Verification items for the finished model (mm, model axes). Coordinates: 2 decimals unless noted, no trailing zeros. Order: outer loops, then holes, each group sorted by start corner. A loop starts at its lowest first (then second) coordinate and runs counter-clockwise, first axis right, second up.
Q1. Thickness scan on line 1 (X direction, y = 177.8, z = 1.8); line 2 (Y direction, x = 12.7, z = 0.9); line 3 (Y direction, x = 495.3, z = 2.05). Record the ranges inside material, lowest first.
Q2. Depth check by flat-ended pin: P1, Ø3, axis at x = 57.15, y = 12.7, coming from the -Z side (3 decimals); P2, Ø1.6, axis at x = 207, z = 1.5, coming from the -Y side. Enter the tip coordinate at first touch or a pass-through.
Q3. Cross-section at B-B, the plane z = 1.6. Count the separate pieces of the cut face and the enclosed holes in it, and give its area (3 significant figures).
Q4. Cross-section at C-C, the plane y = 193. Record the boundary of the cut face in (x, z) (3 decimals).
Q5. Cross-section at D-D, the plane x = 223.5. Record the boundary of the cut face in (y, z) (3 decimals), and give its area (3 significant figures).
from build123d import *

# Parameters (mm, degrees)
SKETCH1_W           = 508
SKETCH1_H           = 508
BOSS_EXTRUDE1_DEPTH = 3.175
SKETCH2_R           = 2.54
SKETCH2_W           = 234.95
SKETCH2_H           = 368.3
CUT_EXTRUDE1_DEPTH  = 44.45
SKETCH4_R           = 2.159
CUT_EXTRUDE3_DEPTH  = 719.427505476
SKETCH5_R           = 2.6
CUT_EXTRUDE4_DEPTH  = 719.427505476
SKETCH6_W           = 487.3625
SKETCH6_H           = 76.2
CUT_EXTRUDE5_DEPTH  = 719.427505476


with BuildPart() as part:
    # Sketch1 → Boss-Extrude1 (new body)
    with BuildSketch(Plane.XY):
        with Locations((254, 254)):
            Rectangle(SKETCH1_W, SKETCH1_H)
    extrude(amount=BOSS_EXTRUDE1_DEPTH)

    # Sketch2 → Cut-Extrude1 (cut)
    with BuildSketch(Plane(origin=(0, 0, 0), x_dir=(-1, 0, 0), z_dir=(0, 0, -1))):
        with Locations((-339.725, 45.085)):
            Circle(SKETCH2_R)
        with Locations((-85.725, 45.085)):
            Circle(SKETCH2_R)
        with Locations((-339.725, 75.565)):
            Circle(SKETCH2_R)
        with Locations((-85.725, 75.565)):
            Circle(SKETCH2_R)
        with Locations((-212.725, 184.15)):
            Rectangle(SKETCH2_W, SKETCH2_H)
        Polygon((0, 403.06625), (0, 328.45375), (-20.6375, 328.45375), (-20.6375, 403.06625), (-20.6375, 508), (0, 508), align=None)
    extrude(amount=-CUT_EXTRUDE1_DEPTH, mode=Mode.SUBTRACT)

    # Sketch4 → Cut-Extrude3 (cut, through all)
    with BuildSketch(Plane(origin=(0, 0, 0), x_dir=(-1, 0, 0), z_dir=(0, 0, -1))):
        with Locations((-311.1754, 390.779)):
            Circle(SKETCH4_R)
        with Locations((-277.1394, 390.779)):
            Circle(SKETCH4_R)
        with Locations((-148.3614, 390.779)):
            Circle(SKETCH4_R)
        with Locations((-114.3254, 390.779)):
            Circle(SKETCH4_R)
    extrude(amount=-CUT_EXTRUDE3_DEPTH, mode=Mode.SUBTRACT)

    # Sketch5 → Cut-Extrude4 (cut, through all)
    with BuildSketch(Plane.XY.offset(3.175)):
        with Locations((12.7, 303.05375)):
            Circle(SKETCH5_R)
        with Locations((12.7, 177.8)):
            Circle(SKETCH5_R)
        with Locations((12.7, 38.1)):
            Circle(SKETCH5_R)
        with Locations((495.3, 38.1)):
            Circle(SKETCH5_R)
        with Locations((495.3, 177.8)):
            Circle(SKETCH5_R)
        with Locations((495.3, 303.05375)):
            Circle(SKETCH5_R)
        with Locations((495.3, 469.9)):
            Circle(SKETCH5_R)
        with Locations((57.15, 12.7)):
            Circle(SKETCH5_R)
        with Locations((368.3, 12.7)):
            Circle(SKETCH5_R)
        with Locations((444.5, 12.7)):
            Circle(SKETCH5_R)
        with Locations((33.3375, 495.3)):
            Circle(SKETCH5_R)
        with Locations((469.9, 495.3)):
            Circle(SKETCH5_R)
    extrude(amount=-CUT_EXTRUDE4_DEPTH, mode=Mode.SUBTRACT)

    # Sketch6 → Cut-Extrude5 (cut, through all)
    with BuildSketch(Plane.XY.offset(3.175)):
        with Locations((264.31875, 469.9)):
            Rectangle(SKETCH6_W, SKETCH6_H)
    extrude(amount=-CUT_EXTRUDE5_DEPTH, mode=Mode.SUBTRACT)


solid = part.part
Check values:
1. line 1: x = 0 to 10.1, 15.3 to 95.25, 330.2 to 492.7, 497.9 to 508
1. line 2: y = 0 to 35.5, 40.7 to 175.2, 180.4 to 300.45, 305.65 to 328.45
1. line 3: y = 0 to 35.5, 40.7 to 175.2, 180.4 to 300.45, 305.65 to 431.8
2. P1: passes through
2. P2: stops at y = 368.3
3. separate pieces: 1
3. enclosed holes: 17
3. area: 130,000 mm2
4. outline: (0, 0) - (95.25, 0) - (95.25, 3.175) - (0, 3.175) - close; (330.2, 0) - (508, 0) - (508, 3.175) - (330.2, 3.175) - close
5. outline: (368.3, 0) - (431.8, 0) - (431.8, 3.175) - (368.3, 3.175) - close
5. area: 202 mm2
